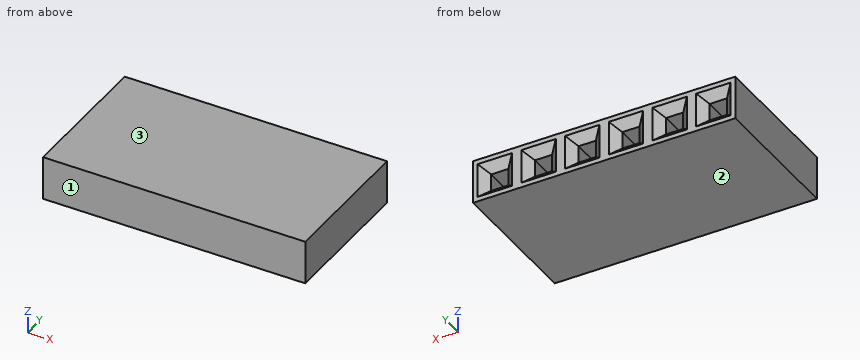
```python
from build123d import *

# Parameters (mm, degrees)
SKETCH1_W                  = 2.54
SKETCH1_H                  = 2.54
BOSS_EXTRUDE1_DEPTH        = 8.3
SKETCH2_W                  = 1
SKETCH2_H                  = 1
CUT_EXTRUDE1_DEPTH         = 4
CHAMFER1_SIZE              = 0.5
LPATTERN1_COUNT            = 6
LPATTERN1_PITCH            = 2.54
CHAMFER1_OF_LPATTERN1_SIZE = 0.5


with BuildPart() as part:
    # Sketch1 → Boss-Extrude1 (new body)
    with BuildSketch(Plane(origin=(0, 0, 0), x_dir=(1, 0, 0), z_dir=(0, 1, 0))):
        Rectangle(SKETCH1_W, SKETCH1_H)
    boss_extrude1 = extrude(amount=BOSS_EXTRUDE1_DEPTH)

    # Sketch2 → Cut-Extrude1 (cut)
    with BuildSketch(Plane(origin=(0, 8.3, 0), x_dir=(-1, 0, 0), z_dir=(0, 1, 0))):
        Rectangle(SKETCH2_W, SKETCH2_H)
    cut_extrude1 = extrude(amount=-CUT_EXTRUDE1_DEPTH, mode=Mode.SUBTRACT)

    # Chamfer1
    chamfer1_edges = [part.edges().sort_by_distance(p)[0] for p in [
        (0, 8.3, 0.5),
        (0.5, 8.3, 0),
        (0, 8.3, -0.5),
        (-0.5, 8.3, 0),
    ]]
    chamfer(chamfer1_edges, length=CHAMFER1_SIZE)

    # LPattern1: Boss-Extrude1, Cut-Extrude1 ×6
    with Locations(*[(i * LPATTERN1_PITCH, 0, 0) for i in range(1, LPATTERN1_COUNT)]):
        add(boss_extrude1)
        add(cut_extrude1, mode=Mode.SUBTRACT)

    # Chamfer1 of LPattern1
    chamfer1_of_lpattern1_edges = [part.edges().sort_by_distance(p)[0] for p in [
        (2.54, 8.3, 0.5),
        (3.04, 8.3, 0),
        (2.54, 8.3, -0.5),
        (2.04, 8.3, 0),
        (5.08, 8.3, 0.5),
        (5.58, 8.3, 0),
        (5.08, 8.3, -0.5),
        (4.58, 8.3, 0),
        (7.62, 8.3, 0.5),
        (8.12, 8.3, 0),
        (7.62, 8.3, -0.5),
        (7.12, 8.3, 0),
        (10.16, 8.3, 0.5),
        (10.66, 8.3, 0),
        (10.16, 8.3, -0.5),
        (9.66, 8.3, 0),
        (12.7, 8.3, 0.5),
        (13.2, 8.3, 0),
        (12.7, 8.3, -0.5),
        (12.2, 8.3, 0),
    ]]
    chamfer(chamfer1_of_lpattern1_edges, length=CHAMFER1_OF_LPATTERN1_SIZE)


solid = part.part
```
CAD build for the part. Positions are in the model's coordinates, mm. Face numbers are marked on the shaded views. Round coordinates to 2 decimals unless told otherwise and drop trailing zeros. Write each loop counter-clockwise with the first axis right and the second up, starting at its lowest first coordinate (ties: lowest second). Pieces come first, ordered by that corner, then holes. Notation, with made-up numbers: (39.25, -35.75) -> (63.25, -35.75) arc R12 ccw to (63.25, -17.75) -> close; hole circle Ø8 at (-30, 39). An arc over 180 degrees is marked (long way). Answer in a Markdown table with one row per item. Add a question column.
Item 1: Saw through at D-D, the plane x = 7.5. Write the cut outline in (y, z), then the cut area to 3 significant figures.
Item 2: Saw through at B-B, the plane z = -0.65. Write the cut outline in (x, y), then the cut area to 3 significant figures.
Item 3: Saw through at A-A, the plane x = 0.75. Write the cut outline in (y, z), then the cut area to 3 significant figures.
Item 4: Mould opens along Z. For the marked faces 1, 2 and 3 say: pulls with the +Z half, pulls with the -Z half, needs draft (parallel to the pull), parting line crosses it, or undercut.
Item 5: Drill centre lines: line 1 (Z direction, x = 2.5, y = 7.5); line 2 (Y direction, x = 5.5, z = 0.15); line 3 (Z direction, x = 3, y = 8.25). Where is each one in solid material? Low to high. Write a range as from..to.
Item 6: Drop flat-ended pins along their axis: pin 1 Ø0.8 at (x, z) = (12.5, 0) entering from +Y; pin 2 Ø0.8 at (x, z) = (0, 0) entering from +Y. Give the stop position or say it passes through.
Item 7: Saw through at C-C, the plane y = 7.5. Write the cut outline in (x, z).
Findings below:
| question | item | result |
|---|---|---|
| 1 | outline | (0, -1.27) -> (8.3, -1.27) -> (8.3, -1) -> (7.8, -0.5) -> (4.3, -0.5) -> (4.3, 0.5) -> (7.8, 0.5) -> (8.3, 1) -> (8.3, 1.27) -> (0, 1.27) -> close |
| 1 | area | 16.8 mm^2 |
| 2 | outline | (-1.27, 0) -> (13.97, 0) -> (13.97, 8.3) -> (13.7, 8.3) -> (13.35, 7.95) -> (12.05, 7.95) -> (11.7, 8.3) -> (11.16, 8.3) -> (10.81, 7.95) -> (9.51, 7.95) -> (9.16, 8.3) -> (8.62, 8.3) -> (8.27, 7.95) -> (6.97, 7.95) -> (6.62, 8.3) -> (6.08, 8.3) -> (5.73, 7.95) -> (4.43, 7.95) -> (4.08, 8.3) -> (3.54, 8.3) -> (3.19, 7.95) -> (1.89, 7.95) -> (1.54, 8.3) -> (1, 8.3) -> (0.65, 7.95) -> (-0.65, 7.95) -> (-1, 8.3) -> (-1.27, 8.3) -> close |
| 2 | area | 123 mm^2 |
| 3 | outline | (0, -1.27) -> (8.3, -1.27) -> (8.3, -1) -> (8.05, -0.75) -> (8.05, 0.75) -> (8.3, 1) -> (8.3, 1.27) -> (0, 1.27) -> close |
| 3 | area | 20.6 mm^2 |
| 4 | face 1 | needs draft |
| 4 | face 2 | pulls with the -Z half |
| 4 | face 3 | pulls with the +Z half |
| 5 | line 1 | z = -1.27..-0.5, 0.5..1.27 |
| 5 | line 2 | y = 0..4.3 |
| 5 | line 3 | z = -1.27..-0.95, 0.95..1.27 |
| 6 | pin 1 | stops at y = 7.9 |
| 6 | pin 2 | stops at y = 4.3 |
| 7 | outline | (-1.27, -1.27) -> (13.97, -1.27) -> (13.97, 1.27) -> (-1.27, 1.27) -> close; hole (-0.5, -0.5) -> (0.5, -0.5) -> (0.5, 0.5) -> (-0.5, 0.5) -> close; hole (2.04, -0.5) -> (3.04, -0.5) -> (3.04, 0.5) -> (2.04, 0.5) -> close; hole (4.58, -0.5) -> (5.58, -0.5) -> (5.58, 0.5) -> (4.58, 0.5) -> close; hole (7.12, -0.5) -> (8.12, -0.5) -> (8.12, 0.5) -> (7.12, 0.5) -> close; hole (9.66, -0.5) -> (10.66, -0.5) -> (10.66, 0.5) -> (9.66, 0.5) -> close; hole (12.2, -0.5) -> (13.2, -0.5) -> (13.2, 0.5) -> (12.2, 0.5) -> close |
